Check sheet for the modelled part. Datum: model origin and axes. Units: mm. Give positions to 0.01 mm unless a question says otherwise; leave off trailing zeros. Order: outer loops, then holes, each group sorted by start corner. A loop starts at its lowest first (then second) coordinate and runs counter-clockwise, first axis right, second up.
from build123d import *

# Parameters (mm, degrees)
F0_W     = 102.730258709
F0_H     = 102.730258709
F0_H_2   = 308.1907761271
F0_H_3   = 154.0953880636
F1_DEPTH = 25.4


# Not quite as in the source:
# - a feature names something its author has since deleted; it is built from what else it names


with BuildPart() as f1:
    # F0 (on Front) → F1 (new body)
    with BuildSketch(Plane.XZ):
        with Locations((-770.1755237305, 217.3844415066)):
            Rectangle(F0_W, F0_H)
        with Locations((-770.1755237305, 11.9239240885)):
            Rectangle(F0_W, F0_H_2)
        with Locations((-770.1755237305, -193.5365933296)):
            Rectangle(F0_W, F0_H)
        with Locations((-770.1755237305, -321.9494167159)):
            Rectangle(F0_W, F0_H_3)
        with Locations((-564.7150063124, -193.5365933296)):
            Rectangle(F0_W, F0_H)
        with Locations((-564.7150063124, 11.9239240885)):
            Rectangle(F0_W, F0_H_2)
        with Locations((-564.7150063124, 217.3844415066)):
            Rectangle(F0_W, F0_H)
        with Locations((-359.2544888943, 217.3844415066)):
            Rectangle(F0_W, F0_H)
        with Locations((-359.2544888943, 11.9239240885)):
            Rectangle(F0_W, F0_H_2)
        with Locations((-359.2544888943, -321.9494167159)):
            Rectangle(F0_W, F0_H_3)
        with Locations((-564.7150063124, -321.9494167159)):
            Rectangle(F0_W, F0_H_3)
        with Locations((-359.2544888943, -193.5365933296)):
            Rectangle(F0_W, F0_H)
        with Locations((-153.7939714763, -193.5365933296)):
            Rectangle(F0_W, F0_H)
        with Locations((-153.7939714763, 217.3844415066)):
            Rectangle(F0_W, F0_H)
        with Locations((-153.7939714763, -321.9494167159)):
            Rectangle(F0_W, F0_H_3)
        with Locations((51.6665459418, -321.9494167159)):
            Rectangle(F0_W, F0_H_3)
        with Locations((51.6665459418, -193.5365933296)):
            Rectangle(F0_W, F0_H)
        with Locations((51.6665459418, 11.9239240885)):
            Rectangle(F0_W, F0_H_2)
        with Locations((-153.7939714763, 11.9239240885)):
            Rectangle(F0_W, F0_H_2)
        with Locations((51.6665459418, 217.3844415066)):
            Rectangle(F0_W, F0_H)
        with Locations((257.1270633599, 217.3844415066)):
            Rectangle(F0_W, F0_H)
        with Locations((257.1270633599, 11.9239240885)):
            Rectangle(F0_W, F0_H_2)
        with Locations((257.1270633599, -193.5365933296)):
            Rectangle(F0_W, F0_H)
        with Locations((257.1270633599, -321.9494167159)):
            Rectangle(F0_W, F0_H_3)
        with Locations((-667.4452650214, 217.3844415066)):
            Rectangle(F0_W, F0_H)
        with Locations((-667.4452650214, -193.5365933296)):
            Rectangle(F0_W, F0_H)
        with Locations((-461.9847476034, -193.5365933296)):
            Rectangle(F0_W, F0_H)
        with Locations((-461.9847476034, 217.3844415066)):
            Rectangle(F0_W, F0_H)
        with Locations((-256.5242301853, 217.3844415066)):
            Rectangle(F0_W, F0_H)
        with Locations((-256.5242301853, -193.5365933296)):
            Rectangle(F0_W, F0_H)
        with Locations((-51.0637127672, -193.5365933296)):
            Rectangle(F0_W, F0_H)
        with Locations((-51.0637127672, 217.3844415066)):
            Rectangle(F0_W, F0_H)
        with Locations((154.3968046508, 217.3844415066)):
            Rectangle(F0_W, F0_H)
        with Locations((154.3968046508, -193.5365933296)):
            Rectangle(F0_W, F0_H)
    extrude(amount=F1_DEPTH)


solid = f1.part
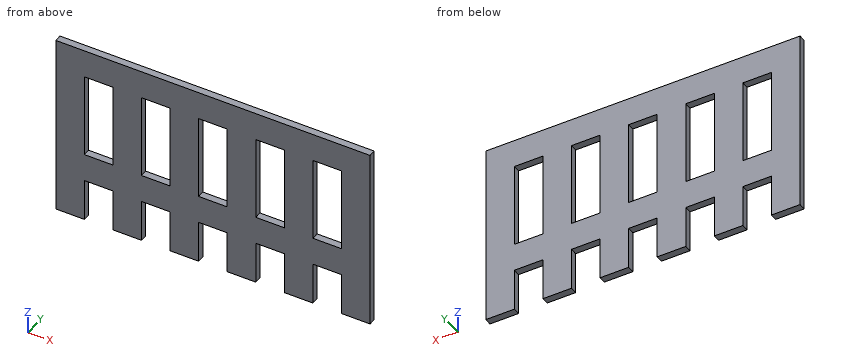
1) Section check A-A, the plane x = -455. Record the cut outline in (y, z).
Recorded:
outline: (-25.4, -244.9) - (0, -244.9) - (0, -142.17) - (-25.4, -142.17) - close; (-25.4, 166.02) - (0, 166.02) - (0, 268.75) - (-25.4, 268.75) - close
2) Section check B-B, the plane z = -29. Record the cut outline in (x, y).
Recorded:
outline: (-821.54, -25.4) - (-718.81, -25.4) - (-718.81, 0) - (-821.54, 0) - close; (-616.08, -25.4) - (-513.35, -25.4) - (-513.35, 0) - (-616.08, 0) - close; (-410.62, -25.4) - (-307.89, -25.4) - (-307.89, 0) - (-410.62, 0) - close; (-205.16, -25.4) - (-102.43, -25.4) - (-102.43, 0) - (-205.16, 0) - close; (0.3, -25.4) - (103.03, -25.4) - (103.03, 0) - (0.3, 0) - close; (205.76, -25.4) - (308.49, -25.4) - (308.49, 0) - (205.76, 0) - close
3) Section check C-C, the plane y = -8.5. State how many separate pieces and enclosed holes the cut face has, then the cut area to 3 significant figures.
Recorded:
separate pieces: 1
enclosed holes: 5
area: 517,000 mm2
4) Depth check by flat-ended pin: pin 1 Ø12.5 at (x, y) = (-646, -14.5) entering from -Z. Enter the tip coordinate at first touch or a pass-through.
Recorded:
pin 1: stops at z = -244.9
5) Material ranges on L1, parallel to X at y = -20.5, z = -32; L2, parallel to Z at x = -659, y = -2, recorded low to high.
Recorded:
L1: x = -821.54 to -718.81, -616.08 to -513.35, -410.62 to -307.89, -205.16 to -102.43, 0.3 to 103.03, 205.76 to 308.49
L2: z = -244.9 to -142.17, 166.02 to 268.75
